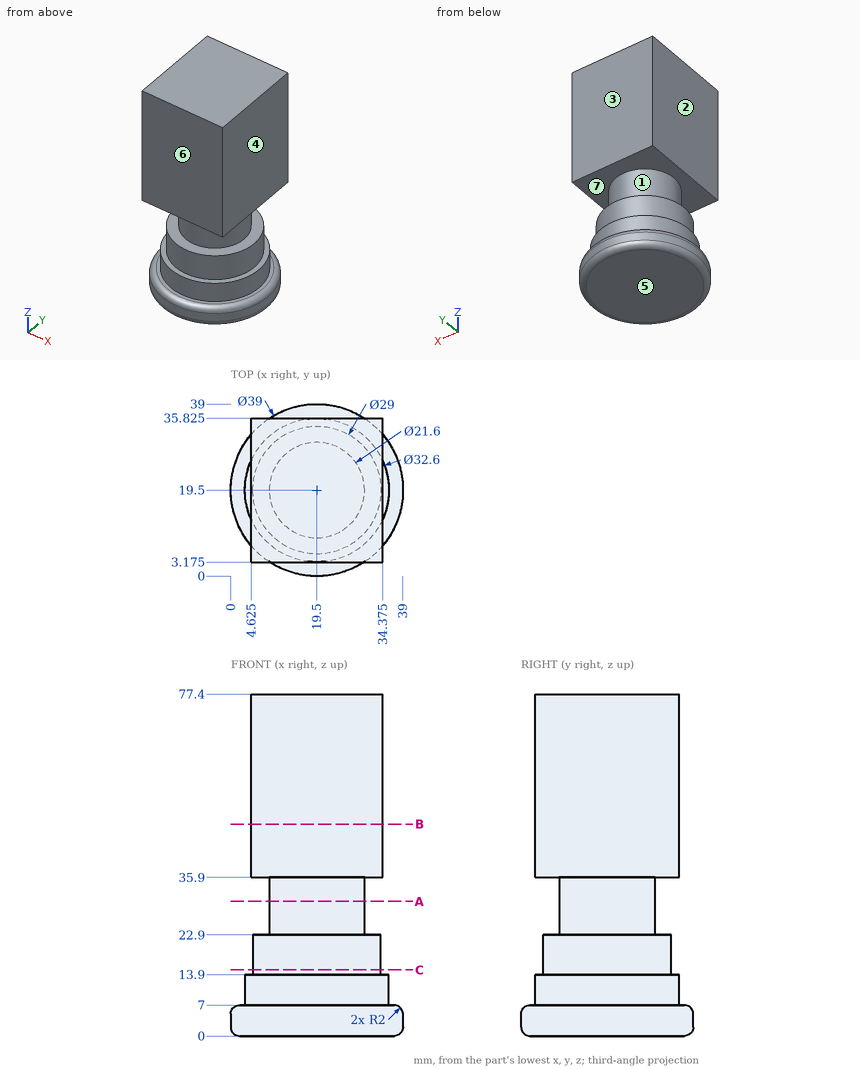
Answer from the drawing. Dimensions are ordinates in mm from the lowest x, y and z of the part. A direction names the side the tool comes from. Coordinates: 2 decimals unless noted, no trailing zeros. Write each loop counter-clockwise with the first axis right and the second up, starting at its lowest first coordinate (ties: lowest second). Pieces come first, ordered by that corner, then holes. Notation, with made-up numbers: (-34, 73.5) - (7, 73.5) arc R23 ccw to (7, 82.5) - close; hole circle Ø7 at (-12.5, -9.75). An arc over 180 degrees is marked (long way). One line per question, with ' | ' between items.
Q1. Find section B-B, the plane z = 48. Write down the section's boundary in (x, y) (3 decimals), plus the area to 3 significant figures.
Result set:
outline: (4.625, 3.175) - (34.375, 3.175) - (34.375, 35.825) - (4.625, 35.825) - close | area: 971 mm^2
Q2. For the marked faces 1, 2, 3 and 4, determine the directions among +Z, -Z, +X, -X, +Y, -Y from which every point of the face is accessible in a straight line to the end or side of a thin tool.
Result set:
face 1: none | face 2: +Z, -X, +Y, -Y | face 3: +Z, +X, -X, +Y | face 4: +Z, +X, +Y, -Y
Q3. Consider L1, parallel to Z at x = 7, y = 27.5; L2, parallel to Z at x = 24, y = 32; L3, parallel to Z at x = 3, y = 26. Determine where each line is inside the solid, lowest interval first. Write a range as [from, to].
Result set:
L1: [0, 13.9], [35.9, 77.4] | L2: [0, 22.9], [35.9, 77.4] | L3: [0.01, 6.99]
Q4. Find section C-C, the plane z = 15. Write down the section's boundary in (x, y), plus the area to 3 significant figures.
Result set:
outline: circle Ø29 at (19.5, 19.5) | area: 661 mm^2
Q5. Find section A-A, the plane z = 30.5. Write down the section's boundary in (x, y), plus the area to 3 significant figures.
Result set:
outline: circle Ø21.6 at (19.5, 19.5) | area: 366 mm^2
Q6. Determine the mould class of the marked faces 5, 6 and 7 for opening direction Z: +Z half, -Z half, draft (parallel to the pull), parting line (faces both ways), or undercut.
Result set:
face 5: -Z half | face 6: draft | face 7: undercut
Q7. Each of these flat-tipped pins is pushed along its axis until it touches: P1, Ø10, axis at x = 33.5, z = 32.5, coming from the +Y side (3 decimals); P2, Ø10, axis at x = 16, z = 61.5, coming from the -Y side (3 decimals); P3, Ø10, axis at y = 33, z = 43.5, coming from the -X side (3 decimals). Where does it stop, or does it pass through?
Result set:
P1: y = 35.825 | P2: y = 3.175 | P3: x = 4.625
